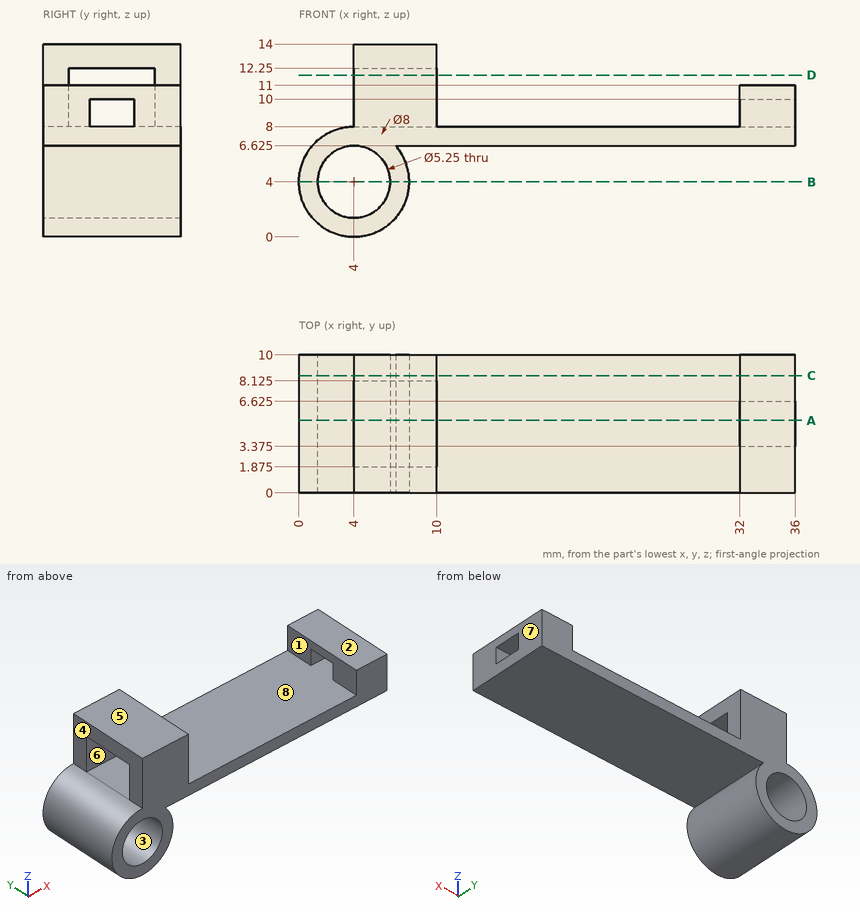
Job drawing, mm, ordinate dimensions from the low corner. One solid piece. A direction names the side the tool comes from. Give positions to 0.01 mm unless a question says otherwise; leave off trailing zeros. Order: outer loops, then holes, each group sorted by start corner. A loop starts at its lowest first (then second) coordinate and runs counter-clockwise, first axis right, second up. Notation, with made-up numbers: M -2,69 L 55,69 A23 cw 55,108 Z; hole C -38,-39.5 d11. An arc over 180 degrees is marked long. Return JSON: item names as keys, results as strings.
Q1. Two-plate mould, pull along Z, no slides. Class the marked faces 5, 6, 7 and 8: pulls with the +Z half, pulls with the -Z half, needs draft (parallel to the pull), parting line crosses it, or undercut.
Answer list:
{"face 5": "pulls with the +Z half", "face 6": "undercut", "face 7": "needs draft", "face 8": "undercut"}
Q2. Wall check: probe 1 along Z at (x, y) = (32.5, 6) (3 decimals); probe 2 along X at (y, z) = (0.5, 4) (3 decimals); probe 3 along Z at (x, y) = (21, 9.75) (3 decimals). Give the ranges that are in metal, low to high. Write a range as from..to.
Answer list:
{"probe 1": "z = 6.625..8, 10..11", "probe 2": "x = 0..1.375, 6.625..8", "probe 3": "z = 6.625..8"}
Q3. 3-axis set-ups, long thin cutter, end or side, ignore diameter. For the marked faces 1, 2, 3 and 4: which of +Z, -Z, +X, -X, +Y, -Y reach the whole face in a straight line?
Answer list:
{"face 1": "+Z, +Y, -Y", "face 2": "+Z, +X, +Y, -Y", "face 3": "+Y, -Y", "face 4": "+Z, -X, +Y, -Y"}
Q4. Band-saw the part on A-A (y = 5.25). Give the cut face in (x, z) (3 decimals), then the cut area to 3 significant figures.
Answer list:
{"outline": "M 4,8 A4 ccw long 7.018,6.625 L 36,6.625 L 36,8 Z; M 4,12.25 L 10,12.25 L 10,14 L 4,14 Z; M 32,10 L 36,10 L 36,11 L 32,11 Z; hole C 4,4 d5.25", "area": "84.2 mm^2"}
Q5. Band-saw the part on D-D (z = 11.75). Give the cut face in (x, y) (3 decimals), then the cut area to 3 significant figures.
Answer list:
{"outline": "M 4,0 L 10,0 L 10,1.875 L 4,1.875 Z; M 4,8.125 L 10,8.125 L 10,10 L 4,10 Z", "area": "22.5 mm^2"}
Q6. Band-saw the part on C-C (y = 8.5). Give the cut face in (x, z) (3 decimals).
Answer list:
{"outline": "M 4,8 A4 ccw long 7.018,6.625 L 36,6.625 L 36,11 L 32,11 L 32,8 L 10,8 L 10,14 L 4,14 Z; hole C 4,4 d5.25"}
Q7. Band-saw the part on B-B (z = 4). Give the cut face in (x, y) (3 decimals), then the cut area to 3 significant figures.
Answer list:
{"outline": "M 0,0 L 1.375,0 L 1.375,10 L 0,10 Z; M 6.625,0 L 8,0 L 8,10 L 6.625,10 Z", "area": "27.5 mm^2"}
Q8. Flat gauge pins, fed straight in: pin 1 (5 mm diameter, centred on x = 23.5, y = 4.5, fed in from +Z); pin 2 (3 mm diameter, centred on y = 4, z = 12.5, fed in from -X); pin 3 (5 mm diameter, centred on x = 15, y = 5.5, fed in from -Z) (3 decimals); pin 4 (3 mm diameter, centred on x = 4, z = 4, fed in from +Y). Where does each tip first touch, or does it go through?
Answer list:
{"pin 1": "stops at z = 8", "pin 2": "stops at x = 4", "pin 3": "stops at z = 6.625", "pin 4": "passes through"}
